Source: three-view drawing plus pictorial views. Frame: mm from the lowest corner of the part. A direction names the side the tool comes from. Give positions to 0.01 mm unless a question says otherwise; leave off trailing zeros. Loops run counter-clockwise (first coordinate to the right, second up) from the corner with the lowest first, then second, coordinate; pieces in that order, holes last. Notation, with made-up numbers: M -18.75,-26.75 L 19.25,-26.75 A16 cw 19.25,-19.75 Z; hole C 25,-24.75 d8. An arc over 180 degrees is marked long. Write item = value, one per line.
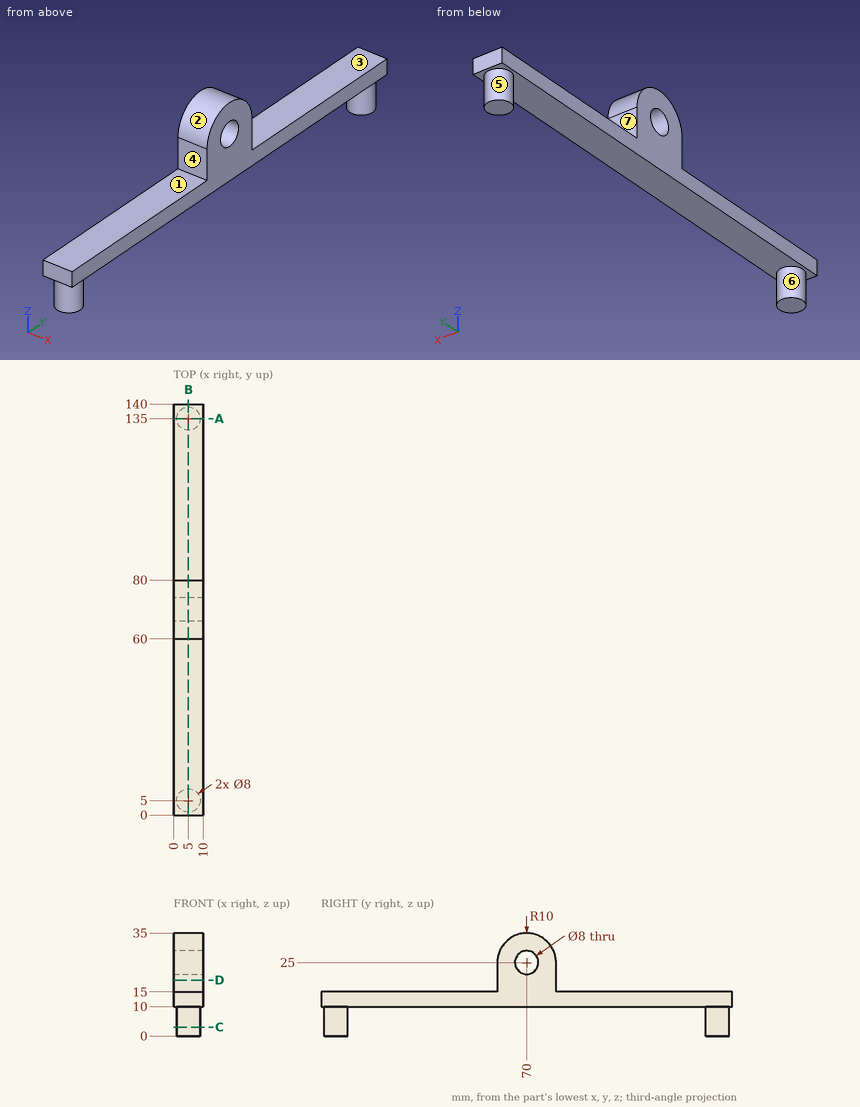
1. First-contact query: pin 1 Ø3 at (x, y) = (3, 72) entering from -Z; pin 2 Ø1.5 at (x, z) = (3, 28.5) entering from +Y; pin 3 Ø3 at (x, z) = (3.5, 20) entering from -Y. Flat tips, straight axial feed; report the tip coordinate or a pass-through.
Derived:
pin_1 = 10
pin_2 = 79.61
pin_3 = 60
2. Cut plane A-A, the plane y = 135. Return the cut outline in (x, z).
Derived:
outline = M 0,10 L 1,10 L 1,0 L 9,0 L 9,10 L 10,10 L 10,15 L 0,15 Z
3. Material intervals for probe 1 along Y at (x, z) = (5.75, 25); probe 2 along Z at (x, y) = (3.5, 100.5); probe 3 along Z at (x, y) = (3.5, 68.5), sorted ascending. Write a range as from..to.
Derived:
probe_1 = 60..66, 74..80
probe_2 = 10..15
probe_3 = 10..21.29, 28.71..34.89
4. Pull-direction query (Y, two-part tool) for the marked faces 4, 5, 6 and 7; classes: +Y half, -Y half, draft (parallel to the pull), parting line (faces both ways), or undercut.
Derived:
face_4 = -Y half
face_5 = undercut
face_6 = undercut
face_7 = +Y half
5. Reachability of the marked faces 1, 2 and 3 from +Z, -Z, +X, -X, +Y, -Y: full face, straight path, thin tool, end or side. Return the list, or none.
Derived:
face_1 = +Z, +X, -X, -Y
face_2 = +Z, +X, -X
face_3 = +Z, +X, -X, +Y
6. Cut plane D-D, the plane z = 19. Return the cut outline in (x, y), then the cut area to 3 significant figures.
Derived:
outline = M 0,60 L 10,60 L 10,80 L 0,80 Z
area = 200 mm²
7. Cut plane B-B, the plane x = 5. Return the cut outline in (y, z), then the cut area to 3 significant figures.
Derived:
outline = M 0,10 L 1,10 L 1,0 L 9,0 L 9,10 L 131,10 L 131,0 L 139,0 L 139,10 L 140,10 L 140,15 L 80,15 L 80,25 A10 ccw 60,25 L 60,15 L 0,15 Z; hole C 70,25 d8
area = 1,170 mm²
8. Cut plane C-C, the plane z = 3. Return the cut outline in (x, y), then the cut area to 3 significant figures.
Derived:
outline = C 5,5 d8; C 5,135 d8
area = 101 mm²
